Build history of the part. All positions in model axes, mm. A direction names the side the tool comes from. Give positions to 0.01 mm unless a question says otherwise; leave off trailing zeros. Order: outer loops, then holes, each group sorted by start corner. A loop starts at its lowest first (then second) coordinate and runs counter-clockwise, first axis right, second up. Notation, with made-up numbers: (8, -39) - (52, -39) arc R22 ccw to (52, -4) - close; hole circle Ø5 at (-21, -2.75). An arc over 180 degrees is marked (long way). Write each question's results on one line, items separated by ' | '. Start each with the question number.
from build123d import *

# Parameters (mm, degrees)
IZIM1_W                     = 300
IZIM1_H                     = 400
Y_KSEKLIK_EKSTR_ZYON1_DEPTH = 200
BO_ALTMA1_T                 = -4
KES_EKSTR_ZYON1_REACH       = 540.516
IZIM2_R                     = 4
KES_EKSTR_ZYON2_REACH       = 540.516
IZIM4_R                     = 4


with BuildPart() as part:
    # izim1 → Y_kseklik-Ekstr_zyon1 (new body)
    with BuildSketch(Plane.XY):
        with Locations((-150, 200)):
            Rectangle(IZIM1_W, IZIM1_H)
    extrude(amount=Y_KSEKLIK_EKSTR_ZYON1_DEPTH)

    # Bo_altma1
    bo_altma1_openings = [part.faces().sort_by_distance(p)[0] for p in [
        (-150, 200, 200),
    ]]
    offset(amount=BO_ALTMA1_T, openings=bo_altma1_openings, kind=Kind.INTERSECTION)

    # izim2 → Kes-Ekstr_zyon1 (cut, up to next)
    with BuildSketch(Plane(origin=(0, 0, 0), x_dir=(0, 0, -1), z_dir=(1, 0, 0)), mode=Mode.PRIVATE) as kes_ekstr_zyon1_sk1:
        with Locations(Location((-146.25, 340, 0), (0, 0, 90))):
            Circle(IZIM2_R)
    kes_ekstr_zyon1_tool1 = extrude(kes_ekstr_zyon1_sk1.sketch, amount=-KES_EKSTR_ZYON1_REACH, mode=Mode.PRIVATE) & part.part
    # izim2 → Kes-Ekstr_zyon1 (cut, up to next)
    with BuildSketch(Plane(origin=(0, 0, 0), x_dir=(0, 0, -1), z_dir=(1, 0, 0)), mode=Mode.PRIVATE) as kes_ekstr_zyon1_sk2:
        with Locations(Location((-53.75, 340, 0), (0, 0, 90))):
            Circle(IZIM2_R)
    kes_ekstr_zyon1_tool2 = extrude(kes_ekstr_zyon1_sk2.sketch, amount=-KES_EKSTR_ZYON1_REACH, mode=Mode.PRIVATE) & part.part
    # izim2 → Kes-Ekstr_zyon1 (cut, up to next)
    with BuildSketch(Plane(origin=(0, 0, 0), x_dir=(0, 0, -1), z_dir=(1, 0, 0)), mode=Mode.PRIVATE) as kes_ekstr_zyon1_sk3:
        with Locations(Location((-146.25, 247.5, 0), (0, 0, 90))):
            Circle(IZIM2_R)
    kes_ekstr_zyon1_tool3 = extrude(kes_ekstr_zyon1_sk3.sketch, amount=-KES_EKSTR_ZYON1_REACH, mode=Mode.PRIVATE) & part.part
    # izim2 → Kes-Ekstr_zyon1 (cut, up to next)
    with BuildSketch(Plane(origin=(0, 0, 0), x_dir=(0, 0, -1), z_dir=(1, 0, 0)), mode=Mode.PRIVATE) as kes_ekstr_zyon1_sk4:
        with Locations(Location((-53.75, 247.5, 0), (0, 0, 90))):
            Circle(IZIM2_R)
    kes_ekstr_zyon1_tool4 = extrude(kes_ekstr_zyon1_sk4.sketch, amount=-KES_EKSTR_ZYON1_REACH, mode=Mode.PRIVATE) & part.part
    kes_ekstr_zyon1_1 = kes_ekstr_zyon1_tool1.solids().sort_by_distance((0, 340, 146.25))[0]
    add(kes_ekstr_zyon1_1, mode=Mode.SUBTRACT)
    kes_ekstr_zyon1_2 = kes_ekstr_zyon1_tool2.solids().sort_by_distance((0, 340, 53.75))[0]
    add(kes_ekstr_zyon1_2, mode=Mode.SUBTRACT)
    kes_ekstr_zyon1_3 = kes_ekstr_zyon1_tool3.solids().sort_by_distance((0, 247.5, 146.25))[0]
    add(kes_ekstr_zyon1_3, mode=Mode.SUBTRACT)
    kes_ekstr_zyon1_4 = kes_ekstr_zyon1_tool4.solids().sort_by_distance((0, 247.5, 53.75))[0]
    add(kes_ekstr_zyon1_4, mode=Mode.SUBTRACT)
    kes_ekstr_zyon1 = kes_ekstr_zyon1_1 + kes_ekstr_zyon1_2 + kes_ekstr_zyon1_3 + kes_ekstr_zyon1_4  # Kes-Ekstr_zyon1 as one shape, for the pattern or mirror that repeats it

    # Aynalama1: Kes-Ekstr_zyon1 across plane
    add(kes_ekstr_zyon1.mirror(Plane(origin=(-150, 0, 0), x_dir=(0, 0, 1), z_dir=(1, 0, 0))), mode=Mode.SUBTRACT)

    # izim4 → Kes-Ekstr_zyon2 (cut, up to next)
    with BuildSketch(Plane.XZ, mode=Mode.PRIVATE) as kes_ekstr_zyon2_sk1:
        with Locations(Location((-280, 146.25, 0), (0, 0, 270))):
            Circle(IZIM4_R)
    kes_ekstr_zyon2_tool1 = extrude(kes_ekstr_zyon2_sk1.sketch, amount=-KES_EKSTR_ZYON2_REACH, mode=Mode.PRIVATE) & part.part
    # izim4 → Kes-Ekstr_zyon2 (cut, up to next)
    with BuildSketch(Plane.XZ, mode=Mode.PRIVATE) as kes_ekstr_zyon2_sk2:
        with Locations(Location((-280, 53.75, 0), (0, 0, 270))):
            Circle(IZIM4_R)
    kes_ekstr_zyon2_tool2 = extrude(kes_ekstr_zyon2_sk2.sketch, amount=-KES_EKSTR_ZYON2_REACH, mode=Mode.PRIVATE) & part.part
    # izim4 → Kes-Ekstr_zyon2 (cut, up to next)
    with BuildSketch(Plane.XZ, mode=Mode.PRIVATE) as kes_ekstr_zyon2_sk3:
        with Locations(Location((-187.5, 146.25, 0), (0, 0, 270))):
            Circle(IZIM4_R)
    kes_ekstr_zyon2_tool3 = extrude(kes_ekstr_zyon2_sk3.sketch, amount=-KES_EKSTR_ZYON2_REACH, mode=Mode.PRIVATE) & part.part
    # izim4 → Kes-Ekstr_zyon2 (cut, up to next)
    with BuildSketch(Plane.XZ, mode=Mode.PRIVATE) as kes_ekstr_zyon2_sk4:
        with Locations(Location((-187.5, 53.75, 0), (0, 0, 270))):
            Circle(IZIM4_R)
    kes_ekstr_zyon2_tool4 = extrude(kes_ekstr_zyon2_sk4.sketch, amount=-KES_EKSTR_ZYON2_REACH, mode=Mode.PRIVATE) & part.part
    # izim4 → Kes-Ekstr_zyon2 (cut, up to next)
    with BuildSketch(Plane.XZ, mode=Mode.PRIVATE) as kes_ekstr_zyon2_sk5:
        with Locations(Location((-20, 146.25, 0), (0, 0, 90))):
            Circle(IZIM4_R)
    kes_ekstr_zyon2_tool5 = extrude(kes_ekstr_zyon2_sk5.sketch, amount=-KES_EKSTR_ZYON2_REACH, mode=Mode.PRIVATE) & part.part
    # izim4 → Kes-Ekstr_zyon2 (cut, up to next)
    with BuildSketch(Plane.XZ, mode=Mode.PRIVATE) as kes_ekstr_zyon2_sk6:
        with Locations(Location((-20, 53.75, 0), (0, 0, 90))):
            Circle(IZIM4_R)
    kes_ekstr_zyon2_tool6 = extrude(kes_ekstr_zyon2_sk6.sketch, amount=-KES_EKSTR_ZYON2_REACH, mode=Mode.PRIVATE) & part.part
    # izim4 → Kes-Ekstr_zyon2 (cut, up to next)
    with BuildSketch(Plane.XZ, mode=Mode.PRIVATE) as kes_ekstr_zyon2_sk7:
        with Locations(Location((-112.5, 53.75, 0), (0, 0, 90))):
            Circle(IZIM4_R)
    kes_ekstr_zyon2_tool7 = extrude(kes_ekstr_zyon2_sk7.sketch, amount=-KES_EKSTR_ZYON2_REACH, mode=Mode.PRIVATE) & part.part
    # izim4 → Kes-Ekstr_zyon2 (cut, up to next)
    with BuildSketch(Plane.XZ, mode=Mode.PRIVATE) as kes_ekstr_zyon2_sk8:
        with Locations(Location((-112.5, 146.25, 0), (0, 0, 90))):
            Circle(IZIM4_R)
    kes_ekstr_zyon2_tool8 = extrude(kes_ekstr_zyon2_sk8.sketch, amount=-KES_EKSTR_ZYON2_REACH, mode=Mode.PRIVATE) & part.part
    add(kes_ekstr_zyon2_tool1.solids().sort_by_distance((-280, 0, 146.25))[0], mode=Mode.SUBTRACT)
    add(kes_ekstr_zyon2_tool2.solids().sort_by_distance((-280, 0, 53.75))[0], mode=Mode.SUBTRACT)
    add(kes_ekstr_zyon2_tool3.solids().sort_by_distance((-187.5, 0, 146.25))[0], mode=Mode.SUBTRACT)
    add(kes_ekstr_zyon2_tool4.solids().sort_by_distance((-187.5, 0, 53.75))[0], mode=Mode.SUBTRACT)
    add(kes_ekstr_zyon2_tool5.solids().sort_by_distance((-20, 0, 146.25))[0], mode=Mode.SUBTRACT)
    add(kes_ekstr_zyon2_tool6.solids().sort_by_distance((-20, 0, 53.75))[0], mode=Mode.SUBTRACT)
    add(kes_ekstr_zyon2_tool7.solids().sort_by_distance((-112.5, 0, 53.75))[0], mode=Mode.SUBTRACT)
    add(kes_ekstr_zyon2_tool8.solids().sort_by_distance((-112.5, 0, 146.25))[0], mode=Mode.SUBTRACT)


solid = part.part
Item 1: Two-plate mould, pull along X, no slides. Class faces 1 (the flat face through (-296, 197, 101)), 2 (the flat face through (0, 197, 99)), 3 (the flat face through (-152, 203, 0)): +X half, -X half, draft (parallel to the pull), parting line (faces both ways), or undercut.
Item 2: Cut at B-B, the plane x = -89.5. List the corners of the cut face in (y, z), then the cut area to 3 significant figures.
Item 3: Probe line 1 along Z through (x, y) = (-2.3, 247.5); line 2 along X through (y, z) = (2, 53); line 3 along X through (y, z) = (174, 12.5). List the from-to ranges inside material, lowest first. Write a range as from..to.
Item 4: Cut at A-A, the plane z = 133. List the corners of the cut face in (x, y), then the cut area to 3 significant figures.
Item 5: Flat gauge pins, fed straight in: pin 1 Ø10 at (y, z) = (356.5, 23) entering from +X; pin 2 Ø6.5 at (x, z) = (-20, 53.75) entering from -Y; pin 3 Ø6 at (x, y) = (-167, 280) entering from +Z; pin 4 Ø6.5 at (y, z) = (340, 146.25) entering from +X (3 decimals). Where does each tip first touch, or does it go through?
Item 6: Which spindle directions (+Z, -Z, +X, -X, +Y, -Y) get a long thin tool onto all of the face, cutting with end or side? Do faces 4 (the flat face through (-300, 197, 99)), 5 (the flat face through (-152, 203, 4)). Say none if no direction does.
Item 7: Cut at C-C, the plane y = 195. List the corners of the cut face in (x, z).
Values found:
1) face 1: undercut | face 2: +X half | face 3: draft
2) outline: (0, 0) - (400, 0) - (400, 200) - (396, 200) - (396, 4) - (4, 4) - (4, 200) - (0, 200) - close | area: 3,170 mm2
3) line 1: z = 0..49.75, 57.75..142.25, 150.25..200 | line 2: x = -300..-283.93, -276.07..-191.43, -183.57..-116.43, -108.57..-23.93, -16.07..0 | line 3: x = -300..-296, -4..0
4) outline: (-300, 0) - (0, 0) - (0, 400) - (-300, 400) - close; hole (-296, 4) - (-4, 4) - (-4, 396) - (-296, 396) - close | area: 5,540 mm2
5) pin 1: stops at x = 0 | pin 2: stops at y = 396 | pin 3: stops at z = 4 | pin 4: passes through
6) face 4: +Z, -Z, -X, +Y, -Y | face 5: +Z
7) outline: (-300, 0) - (0, 0) - (0, 200) - (-4, 200) - (-4, 4) - (-296, 4) - (-296, 200) - (-300, 200) - close
